Build history of the part. All positions in model axes, mm. Give positions to 0.01 mm unless a question says otherwise; leave off trailing zeros. Order: outer loops, then holes, each group sorted by start corner. A loop starts at its lowest first (then second) coordinate and runs counter-clockwise, first axis right, second up. Notation, with made-up numbers: M 15,86 L 20,86 A17 cw 20,116 Z; hole C 49,-37 d3. An arc over 180 degrees is marked long. One line per item, written item: value.
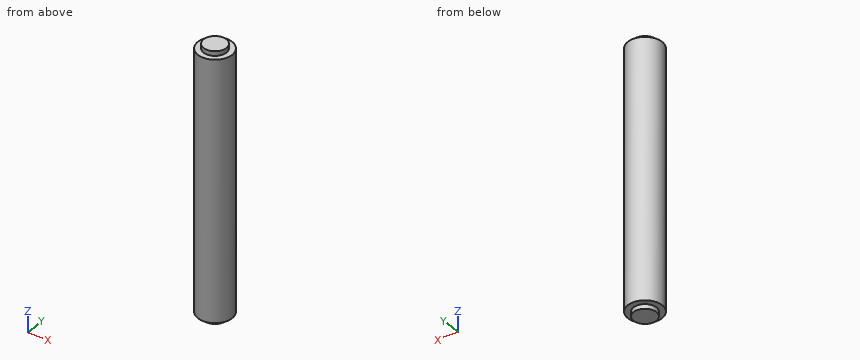
Autodesk Inventor part; units mm, degrees
ref_plane "YZ Plane" through (0, 0, 0) normal (1, 0, 0) x (0, 1, 0)
ref_plane "XZ Plane" through (0, 0, 0) normal (0, 1, 0) x (-1, 0, 0)
ref_plane "XY Plane" through (0, 0, 0) normal (0, 0, 1) x (1, 0, 0)
sketch "Skizze1" plane through (0, 0, 0) normal (0, 0, 1) x (1, 0, 0)
  circle A0 centre (0, 0) radius 22.5
  dimension "d0" = 45
extrude "Extrusion1" add sketch "Skizze1" along normal blind 338
sketch "Skizze2" plane through (0, 0, 338) normal (0, 0, 1) x (1, 0, 0)
  point P0 (0, 0)
sketch "Skizze3" plane through (0, 0, 338) normal (0, 0, 1) x (1, 0, 0)
  circle A0 centre (0, 0) radius 15
  dimension "d3" = 30
extrude "Extrusion2" add sketch "Skizze3" along normal blind 6
sketch "Skizze4" plane through (0, 0, 0) normal (0, 0, -1) x (-1, 0, 0)
  circle A0 centre (0, 0) radius 15
extrude "Extrusion3" add sketch "Skizze4" along normal blind 6
properties part number "Welle"
1) Saw through at A-A, the plane z = 32. Write the cut outline in (x, y), then the cut area to 3 significant figures.
Check values:
outline: C 0,0 d45
area: 1,590 mm^2
2) Saw through at C-C, the plane y = -18. Write the cut outline in (x, z), then the cut area to 3 significant figures.
Check values:
outline: M -13.5,0 L 13.5,0 L 13.5,338 L -13.5,338 Z
area: 9,130 mm^2
3) Pin check, flat tips, straight feed: pin 1 (6 mm diameter, centred on y = -4, z = 239, fed in from -X); pin 2 (6 mm diameter, centred on y = -11.5, z = 169, fed in from +X); pin 3 (1 mm diameter, centred on x = 13.5, z = 236, fed in from -Y). Stop position of each tip, or through.
Check values:
pin 1: x = -22.48
pin 2: x = 20.83
pin 3: y = -18.36
4) Drill centre lines: probe 1 along Z at (x, y) = (15.5, -2); probe 2 along Y at (x, z) = (-4, 235); probe 3 along X at (y, z) = (-7, 157.5). Where is each one in solid material? Low to high. Write a range as from..to.
Check values:
probe 1: 0..338
probe 2: -22.14..22.14
probe 3: -21.38..21.38
5) Saw through at B-B, the plane x = -9. Write the cut outline in (y, z).
Check values:
outline: M -20.62,0 L -12,0 L -12,-6 L 12,-6 L 12,0 L 20.62,0 L 20.62,338 L 12,338 L 12,344 L -12,344 L -12,338 L -20.62,338 Z
